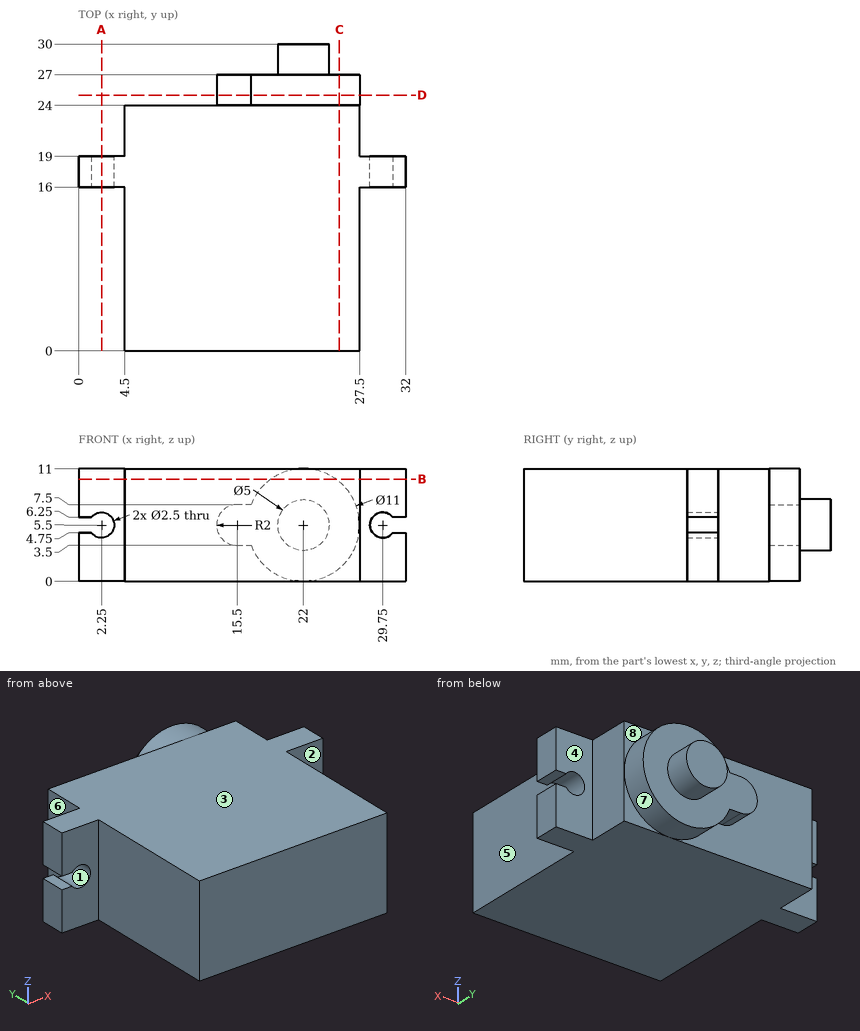
Verification items for this drawing (mm, ordinates from the low corner). A direction names the side the tool comes from. Coordinates: 2 decimals unless noted, no trailing zeros. Write each loop counter-clockwise with the first axis right and the second up, starting at its lowest first coordinate (ties: lowest second). Pieces come first, ordered by that corner, then holes. Notation, with made-up numbers: M -22,6 L -2,6 A28 ccw -2,35 Z; hole C 36,86.25 d7. An arc over 180 degrees is marked long. Answer as a JSON object with one key per item and string values.
1. Section check B-B, the plane z = 10. Enter the section's corners in (x, y), plus the area to 3 significant figures.
Answers below:
{"outline": "M 0,16 L 4.5,16 L 4.5,0 L 27.5,0 L 27.5,16 L 32,16 L 32,19 L 27.5,19 L 27.5,24 L 25.16,24 L 25.16,27 L 18.84,27 L 18.84,24 L 4.5,24 L 4.5,19 L 0,19 Z", "area": "598 mm²"}
2. Section check C-C, the plane x = 25.5. Enter the section's corners in (y, z).
Answers below:
{"outline": "M 0,0 L 24,0 L 24,1.26 L 27,1.26 L 27,9.74 L 24,9.74 L 24,11 L 0,11 Z"}
3. Draft check along Z on the marked faces 1, 2 and 3. Enter one of: released by +Z, released by -Z, zero draft, split by the parting line, or undercut.
Answers below:
{"face 1": "undercut", "face 2": "zero draft", "face 3": "released by +Z"}
4. Go/stop test with flat-tipped pins: pin 1 Ø1.1 at (x, y) = (16.5, 25.5) entering from +Z; pin 2 Ø3 at (y, z) = (26.5, 9.5) entering from +X; pin 3 Ø3.5 at (y, z) = (8, 5) entering from -X. Record where each tip stops, or that it passes through.
Answers below:
{"pin 1": "stops at z = 7.9", "pin 2": "stops at x = 26.9", "pin 3": "stops at x = 4.5"}
5. Section check D-D, the plane y = 25. Enter the section's corners in (x, z), plus the area to 3 significant figures.
Answers below:
{"outline": "M 15.5,3.5 L 16.88,3.5 A5.5 ccw long 16.88,7.5 L 15.5,7.5 A2 ccw Z", "area": "106 mm²"}
6. Tool access check on the marked faces 4, 5, 6, 7 and 8. Record the directions out of +Z, -Z, +X, -X, +Y, -Y that give a thin tool (end or side, any length) a straight path to the whole face; none if there is none.
Answers below:
{"face 4": "+Z, -Z, +X, +Y", "face 5": "+Z, -Z, +X, -Y", "face 6": "+Z, -Z, -X, +Y", "face 7": "+Y", "face 8": "+Z, +X, +Y"}
7. Scan lines: L1, parallel to Z at x = 2.25, y = 18.05; L2, parallel to X at y = 21.5, z = 7; L3, parallel to Y at x = 7.5, z = 10.25. Record each from-to range of solid material in increasing order.
Answers below:
{"L1": "z = 0 to 4.25, 6.75 to 11", "L2": "x = 4.5 to 27.5", "L3": "y = 0 to 24"}
8. Section check A-A, the plane x = 2.25. Enter the section's corners in (y, z), plus the area to 3 significant figures.
Answers below:
{"outline": "M 16,0 L 19,0 L 19,4.25 L 16,4.25 Z; M 16,6.75 L 19,6.75 L 19,11 L 16,11 Z", "area": "25.5 mm²"}
